Check sheet for the modelled part. Datum: model origin and axes. Units: mm. Face numbers are marked on the shaded views. A direction names the side the tool comes from. Give positions to 0.01 mm unless a question says otherwise; leave off trailing zeros. Loops run counter-clockwise (first coordinate to the right, second up) from the corner with the lowest first, then second, coordinate; pieces in that order, holes last. Notation, with made-up numbers: (38.5, 73) -> (90.5, 73) arc R27 ccw to (90.5, 95) -> close; hole circle Ø1 at (-10.5, 22.5). An arc over 180 degrees is marked (long way). Write each question's results on one line, items separated by ' | '. Start each with the question number.
Item 1: Gauge pin test, flat ends, axial feed: pin 1 Ø7.5 at (x, y) = (51, 3.5) entering from +Z; pin 2 Ø1 at (y, z) = (15.5, 0) entering from +X. Record the tip position at first contact, or that the pin passes through.
Item 2: Scan lines: line 1 along X through (y, z) = (0.5, -0.5); line 2 along X through (y, z) = (-18, -2.5); line 3 along Y through (x, z) = (-37, 1.5). Record each from-to range of solid material in increasing order.
Item 3: Mould release check, pull along Y, two halves, no side actions. Record for the marked faces 3, 4 and 5: pulls with the +Y half, pulls with the -Y half, needs draft (parallel to the pull), parting line crosses it, or undercut.
Item 4: Access from +Z, -Z, +X, -X, +Y, -Y to the whole of each face (thin tool, end or side, straight path). Record for the marked faces 1 and 2.
Item 5: Cross-section at A-A on y = -25. Enter the section's corners in (x, z), then the cut area to 3 significant figures.
Item 6: Cross-section at B-B on x = 39. Enter the section's corners in (y, z).
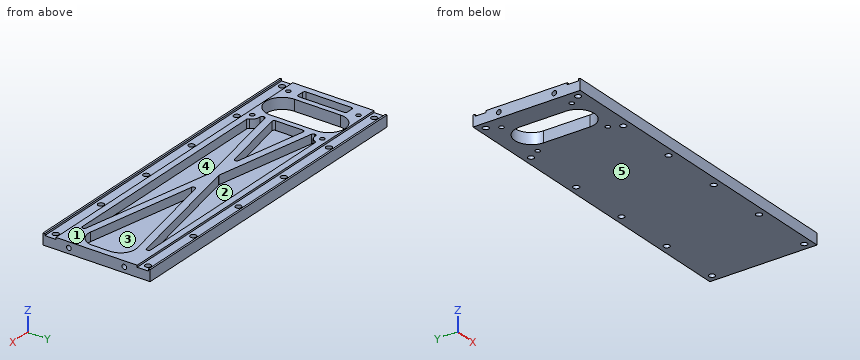
from build123d import *

# Parameters (mm, degrees)
SKETCH_1_W               = 177
SKETCH_1_H               = 58
EXTRUDE_1_DEPTH          = 3
CUT_EXTRUDE_START        = 3
SKETCH_1_3_W             = 177
SKETCH_1_3_H             = 6
CUT_EXTRUDE_1_DEPTH      = 1
CUT_EXTRUDE_2_DEPTH      = 94.178591962
CUT_EXTRUDE_2_DEPTH_BACK = 94.178591962
HOLE_WIZARD_M3_1_D       = 3.2
M3X0_5_2_D               = 2.5
M3X0_5_2_ON_FACE_2_D     = 2.5
CUT_EXTRUDE_5_DEPTH      = 4.8
FILLET_4_R               = 8
FILLET_5_R               = 1.1
M3X0_5_1_D               = 2.5
M3X0_5_1_DEPTH           = 8.5
M3X0_5_1_TIP             = 0.751075774
M3X0_5_1_ON_FACE_2_D     = 2.5
M3X0_5_1_ON_FACE_2_DEPTH = 8.5
M3X0_5_1_ON_FACE_2_TIP   = 0.751075774


with BuildPart() as part:
    # ｽｹｯﾁ1 → ﾎﾞｽ - 押し出し1 (new, symmetric)
    with BuildSketch(Plane.XY):
        Rectangle(SKETCH_1_W, SKETCH_1_H)
    extrude(amount=EXTRUDE_1_DEPTH, both=True)

    # ｽｹｯﾁ1<3> → ｶｯﾄ - 押し出し1 (cut)
    with BuildSketch(Plane.XY.offset(CUT_EXTRUDE_START)):
        with Locations((0, -25)):
            Rectangle(SKETCH_1_3_W, SKETCH_1_3_H)
        with Locations((0, 25)):
            Rectangle(SKETCH_1_3_W, SKETCH_1_3_H)
    extrude(amount=-CUT_EXTRUDE_1_DEPTH, mode=Mode.SUBTRACT)

    # ｽｹｯﾁ1<4> → ｶｯﾄ - 押し出し2 (cut, two sides: drawn at the far end of the back side and taken through both)
    with BuildSketch(Plane.XY.offset(-CUT_EXTRUDE_2_DEPTH_BACK)):
        with BuildLine():
            Line((-58.5, 12.5), (-58.5, -12.5))
            ThreePointArc((-58.5, -12.5), (-67.5, -21.5), (-76.5, -12.5))
            Line((-76.5, -12.5), (-76.5, 12.5))
            ThreePointArc((-76.5, 12.5), (-67.5, 21.5), (-58.5, 12.5))
        make_face()
    extrude(amount=CUT_EXTRUDE_2_DEPTH + CUT_EXTRUDE_2_DEPTH_BACK, mode=Mode.SUBTRACT)

    # M3 すきま穴1 (through all)
    with Locations(Plane(origin=(-84.5, -25, -3), x_dir=(-1, 0, 0), z_dir=(0, 0, -1))):
        with Locations((0, 0), (-33.8, 0), (-67.6, 0), (-101.4, 0), (-135.2, 0), (-169, 0), (-169, 50), (-135.2, 50), (-101.4, 50), (-67.6, 50), (-33.8, 50), (0, 50)):
            Hole(HOLE_WIZARD_M3_1_D / 2)

    # M3x0.5 ねじ穴2 (through all)
    with Locations(Plane(origin=(-81, 19, 3), x_dir=(1, 0, 0), z_dir=(0, 0, 1))):
        with Locations((0, 0), (0, -38), (27, -38)):
            Hole(M3X0_5_2_D / 2)

    # M3x0.5 ねじ穴2 on face 2 (through all)
    with Locations(Plane(origin=(-54, 19, -3), x_dir=(-1, 0, 0), z_dir=(0, 0, -1))):
        with Locations((0, 0)):
            Hole(M3X0_5_2_ON_FACE_2_D / 2)

    # ｽｹｯﾁ12 → ｶｯﾄ - 押し出し5 (cut)
    with BuildSketch(Plane.XY.offset(3)):
        with BuildLine():
            Line((-85, 13.354524038), (-85, -13.354524038))
            Line((-85, -13.354524038), (-79.469535859, -13.354524038))
            ThreePointArc((-79.469535859, -13.354524038), (-79.492381546, -12.927533448), (-79.5, -12.5))
            Line((-79.5, -12.5), (-79.5, 12.5))
            ThreePointArc((-79.5, 12.5), (-79.492381546, 12.927533448), (-79.469535859, 13.354524038))
            Line((-79.469535859, 13.354524038), (-85, 13.354524038))
        make_face()
        with BuildLine():
            Line((-50.031373033, -18.5), (85, -18.5))
            Line((85, -18.5), (0, -2.037166752))
            Line((0, -2.037166752), (-55.503434775, -12.78709371))
            ThreePointArc((-55.503434775, -12.78709371), (-55.612117039, -14.136532524), (-55.872105383, -15.46514195))
            ThreePointArc((-55.872105383, -15.46514195), (-52.155700259, -15.450555189), (-50.031373033, -18.5))
        make_face()
        Polygon((85, -14.425666496), (85, 14.425666496), (10.518187928, 0), align=None)
        with BuildLine():
            Line((85, 18.5), (-50.031373033, 18.5))
            ThreePointArc((-50.031373033, 18.5), (-52.155700259, 15.450555189), (-55.872105383, 15.46514195))
            ThreePointArc((-55.872105383, 15.46514195), (-55.612117039, 14.136532524), (-55.503434775, 12.78709371))
            Line((-55.503434775, 12.78709371), (0, 2.037166752))
            Line((0, 2.037166752), (85, 18.5))
        make_face()
        Polygon((-55.5, -8.712094957), (-55.5, 8.712094957), (-10.518187928, 0), align=None)
    extrude(amount=-CUT_EXTRUDE_5_DEPTH, mode=Mode.SUBTRACT)

    # ﾌｨﾚｯﾄ4
    fillet_4_edges = [part.edges().sort_by_distance(p)[0] for p in [
        (85, -14.425666496, 0.6),
        (85, 14.425666496, 0.6),
    ]]
    fillet(fillet_4_edges, radius=FILLET_4_R)

    # ﾌｨﾚｯﾄ5
    fillet_5_edges = [part.edges().sort_by_distance(p)[0] for p in [
        (85, -18.5, 0.6),
        (0, -2.037166752, 0.6),
        (-55.503434775, -12.78709371, 0.6),
        (-55.872105383, -15.46514195, 0.6),
        (-50.031373033, -18.5, 0.6),
        (-50.031373033, 18.5, 0.6),
        (-55.872105383, 15.46514195, 0.6),
        (-55.503434775, 12.78709371, 0.6),
        (0, 2.037166752, 0.6),
        (85, 18.5, 0.6),
        (10.518187928, 0, 0.6),
        (-55.5, -8.712094957, 0.6),
        (-10.518187928, 0, 0.6),
        (-55.5, 8.712094957, 0.6),
        (-85, -13.354524038, 0.6),
        (-79.469535859, -13.354524038, 0.6),
        (-85, 13.354524038, 0.6),
        (-79.469535859, 13.354524038, 0.6),
    ]]
    fillet(fillet_5_edges, radius=FILLET_5_R)

    # M3x0.5 ねじ穴1
    with Locations(Plane(origin=(-88.5, 15, 0), x_dir=(0, 0, -1), z_dir=(-1, 0, 0))):
        with Locations((0, 0), (0, 30)):
            Hole(M3X0_5_1_D / 2, depth=M3X0_5_1_DEPTH)
            with Locations((0, 0, -(M3X0_5_1_DEPTH + M3X0_5_1_TIP / 2))):  # 118° drill point
                Cone(0, M3X0_5_1_D / 2, M3X0_5_1_TIP, mode=Mode.SUBTRACT)

    # M3x0.5 ねじ穴1 on face 2
    with Locations(Plane(origin=(88.5, 15, 0), x_dir=(0, 0, 1), z_dir=(1, 0, 0))):
        with Locations((0, 0), (0, 30)):
            Hole(M3X0_5_1_ON_FACE_2_D / 2, depth=M3X0_5_1_ON_FACE_2_DEPTH)
            with Locations((0, 0, -(M3X0_5_1_ON_FACE_2_DEPTH + M3X0_5_1_ON_FACE_2_TIP / 2))):  # 118° drill point
                Cone(0, M3X0_5_1_ON_FACE_2_D / 2, M3X0_5_1_ON_FACE_2_TIP, mode=Mode.SUBTRACT)


solid = part.part
Answer sheet:
1) pin 1: stops at z = -1.8 | pin 2: stops at x = 79.85
2) line 1: x = -88.5 to -85, -79.5 to -76.5, -58.5 to -55.5, -15.32 to 15.32, 85 to 88.5 | line 2: x = -88.5 to -81.75, -80.25 to -74.62, -60.38 to -54.75, -53.25 to 88.5 | line 3: y = -29 to -18.5, -9.2 to -5.13, 5.13 to 9.2, 18.5 to 29
3) face 3: undercut | face 4: undercut | face 5: needs draft
4) face 1: +Z, +X, -X, +Y, -Y | face 2: +Z
5) outline: (-88.5, -3) -> (-86.1, -3) -> (-86.1, 2) -> (-88.5, 2) -> close; (-82.9, -3) -> (-52.3, -3) -> (-52.3, 2) -> (-82.9, 2) -> close; (-49.1, -3) -> (-18.5, -3) -> (-18.5, 2) -> (-49.1, 2) -> close; (-15.3, -3) -> (15.3, -3) -> (15.3, 2) -> (-15.3, 2) -> close; (18.5, -3) -> (49.1, -3) -> (49.1, 2) -> (18.5, 2) -> close; (52.3, -3) -> (82.9, -3) -> (82.9, 2) -> (52.3, 2) -> close; (86.1, -3) -> (88.5, -3) -> (88.5, 2) -> (86.1, 2) -> close | area: 789 mm²
6) outline: (-29, -3) -> (29, -3) -> (29, 3) -> (28, 3) -> (28, 2) -> (22, 2) -> (22, 3) -> (18.5, 3) -> (18.5, -1.8) -> (9.59, -1.8) -> (9.59, 3) -> (5.52, 3) -> (5.52, -1.8) -> (-5.52, -1.8) -> (-5.52, 3) -> (-9.59, 3) -> (-9.59, -1.8) -> (-18.5, -1.8) -> (-18.5, 3) -> (-22, 3) -> (-22, 2) -> (-28, 2) -> (-28, 3) -> (-29, 3) -> close
